For this review, use the dimensioned drawing (mm, ordinates from the lowest corner) and the shaded views. A direction names the side the tool comes from. Coordinates: 2 decimals unless noted, no trailing zeros. Loops run counter-clockwise (first coordinate to the right, second up) from the corner with the lowest first, then second, coordinate; pieces in that order, holes last. Notation, with made-up numbers: (86, 53) - (145, 53) arc R21 ccw to (145, 63) - close; hole circle Ø4 at (13, -30). An arc over 180 degrees is marked (long way). One line per item, written item: value. Start each with the question number.
1. For the marked faces 1 and 2, list the 3-axis set-ups (+Z, -Z, +X, -X, +Y, -Y) from which the entire face can be reached by the end or side of a thin tool; tool diameter is ignored.
2. We need section D-D, the plane y = 1. Give the boundary of the cut face in (x, z), then the cut area to 3 significant figures.
3. We need section C-C, the plane y = 6.75. Give the boundary of the cut face in (x, z), then the cut area to 3 significant figures.
4. Mouldability with a two-part tool opening along Y and no side actions: class the marked faces 3, 4, 5 and 6 as +Y half, -Y half, draft (parallel to the pull), parting line (faces both ways), or undercut.
5. We need section B-B, the plane z = 2.6. Give the boundary of the cut face in (x, y).
6. To check wall thickness, follow line 1 (Y direction, x = 32, z = 2); line 2 (X direction, y = 5.5, z = 4.45); line 3 (X direction, y = 6, z = 0.5). State the ranges of each line that lie inside material, in increasing order.
7. We need section A-A, the plane x = 19. Give the boundary of the cut face in (y, z).
8. Insertion check: P1, Ø1.5, axis at x = 52, y = 6, coming from the -Z side; P2, Ø1.5, axis at y = 8, z = 3.5, coming from the -X side. Each pin has a flat end and moves straight along its axis. Give the tip position at first contact, or say it passes through.
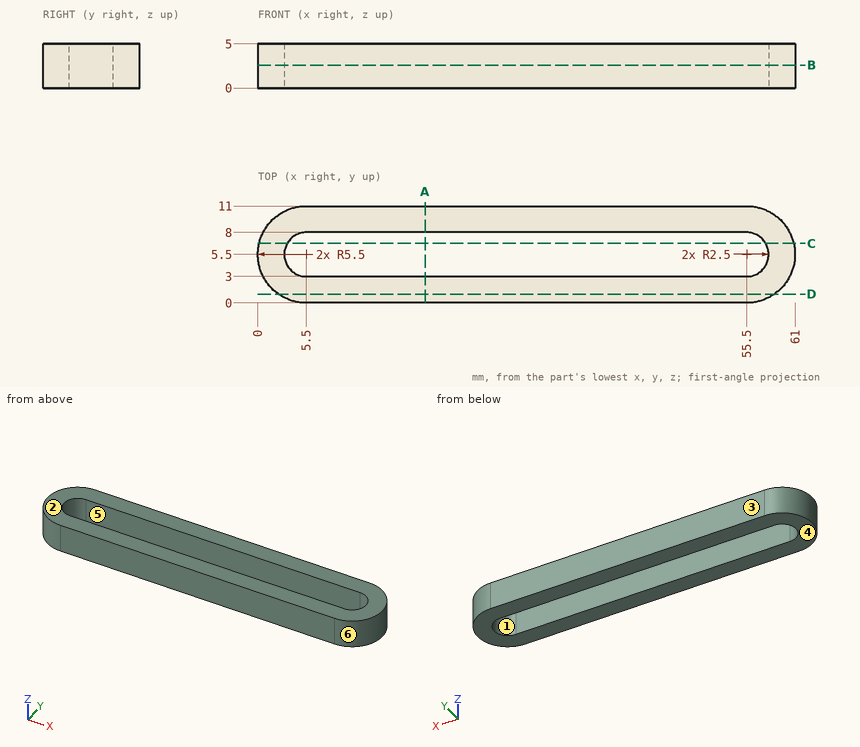
Findings below:
1. face 1: +Z, -Z
1. face 2: +Z, +X, -X, +Y, -Y
2. outline: (2.34, 0) - (58.66, 0) - (58.66, 5) - (2.34, 5) - close
2. area: 282 mm2
3. outline: (0.14, 0) - (3.33, 0) - (3.33, 5) - (0.14, 5) - close; (57.67, 0) - (60.86, 0) - (60.86, 5) - (57.67, 5) - close
3. area: 31.9 mm2
4. face 3: +Y half
4. face 4: draft
4. face 5: undercut
4. face 6: parting line
5. outline: (5.5, 0) - (55.5, 0) arc R5.5 ccw to (55.5, 11) - (5.5, 11) arc R5.5 ccw to start; hole (5.5, 3) - (55.5, 3) arc R2.5 ccw to (55.5, 8) - (5.5, 8) arc R2.5 ccw to start
6. line 1: 0 to 3, 8 to 11
6. line 2: 0 to 3, 58 to 61
6. line 3: 0.02 to 3.05, 57.95 to 60.98
7. outline: (0, 0) - (3, 0) - (3, 5) - (0, 5) - close; (8, 0) - (11, 0) - (11, 5) - (8, 5) - close
8. P1: through
8. P2: x = 0.29
